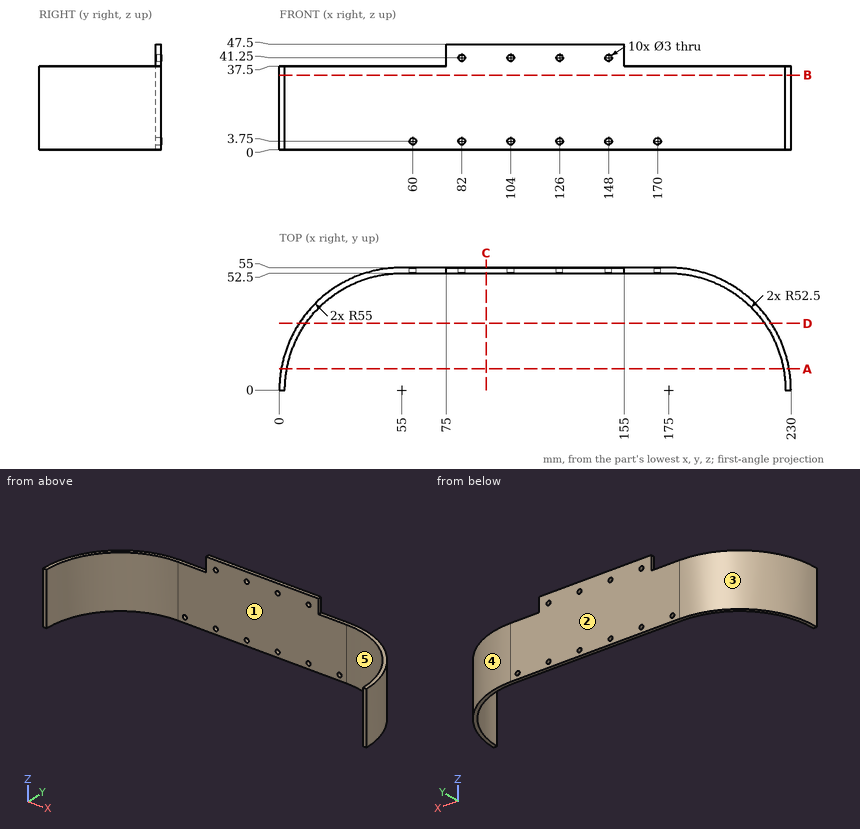
Job drawing, mm, ordinate dimensions from the low corner. One solid piece. A direction names the side the tool comes from. Give positions to 0.01 mm unless a question says otherwise; leave off trailing zeros. Write each loop counter-clockwise with the first axis right and the second up, starting at its lowest first coordinate (ties: lowest second). Pieces come first, ordered by that corner, then holes. Notation, with made-up numbers: (-6, 85.25) - (17, 85.25) arc R28 ccw to (17, 117.25) - close; hole circle Ø11 at (85.25, -13). An arc over 180 degrees is marked (long way). Answer as CSV lines item,"result".
1. 3-axis set-ups, long thin cutter, end or side, ignore diameter. For the marked faces 4 and 5: which of +Z, -Z, +X, -X, +Y, -Y reach the whole face in a straight line?
Responses:
face 4,"+Z, -Z, +X, +Y"
face 5,"+Z, -Z, -Y"
2. Pin check, flat tips, straight feed: pin 1 (5 mm diameter, centred on x = 104, z = 41.25, fed in from -Y); pin 2 (3 mm diameter, centred on y = 53.5, z = 42.5, fed in from -X); pin 3 (2.5 mm diameter, centred on x = 104, z = 3.75, fed in from -Y); pin 4 (1.2 mm diameter, centred on y = 54, z = 44.5, fed in from +X). Stop position of each tip, or through.
Responses:
pin 1,"stops at y = 52.5"
pin 2,"stops at x = 75"
pin 3,"passes through"
pin 4,"stops at x = 155"
3. Two-plate mould, pull along X, no slides. Class the marked faces 1, 2 and 3: +X half, -X half, draft (parallel to the pull), parting line (faces both ways), or undercut.
Responses:
face 1,"undercut"
face 2,"draft"
face 3,"-X half"
4. Band-saw the part on B-B (z = 33.5). Write the cut outline in (x, y), and give its area (3 significant figures).
Responses:
outline,"(0, 0) - (2.5, 0) arc R52.5 cw to (55, 52.5) - (175, 52.5) arc R52.5 cw to (227.5, 0) - (230, 0) arc R55 ccw to (175, 55) - (55, 55) arc R55 ccw to start"
area,"722 mm2"
5. Band-saw the part on C-C (x = 93). Write the cut outline in (y, z).
Responses:
outline,"(52.5, 0) - (55, 0) - (55, 47.5) - (52.5, 47.5) - close"
6. Drill centre lines: L1, parallel to Z at x = 104, y = 53.3; L2, parallel to X at y = 54.45, z = 41.25; L3, parallel to Y at x = 116.5, z = 5. Where is each one in solid material? Low to high. Write a range as [from, to].
Responses:
L1,"z = [0, 2.25], [5.25, 39.75], [42.75, 47.5]"
L2,"x = [75, 80.5], [83.5, 102.5], [105.5, 124.5], [127.5, 146.5], [149.5, 155]"
L3,"y = [52.5, 55]"
7. Band-saw the part on A-A (y = 9.5). Write the cut outline in (x, z), and give its area (3 significant figures).
Responses:
outline,"(0.83, 0) - (3.37, 0) - (3.37, 37.5) - (0.83, 37.5) - close; (226.63, 0) - (229.17, 0) - (229.17, 37.5) - (226.63, 37.5) - close"
area,"191 mm2"
8. Band-saw the part on D-D (y = 30). Write the cut outline in (x, z), and give its area (3 significant figures).
Responses:
outline,"(8.9, 0) - (11.92, 0) - (11.92, 37.5) - (8.9, 37.5) - close; (218.08, 0) - (221.1, 0) - (221.1, 37.5) - (218.08, 37.5) - close"
area,"226 mm2"
